Can you work these out from the model? Positions are in its coordinate system, mm. A direction names the side the tool comes from. Give positions to 0.01 mm unless a question says otherwise; leave off trailing zeros. Loops run counter-clockwise (first coordinate to the right, second up) from the corner with the lowest first, then second, coordinate; pieces in that order, holes last. Notation, with made-up numbers: (80, 36) -> (124, 36) arc R23 ccw to (124, 50) -> close; hole circle Ø10 at (71.5, -18). An arc over 180 degrees is marked (long way). One line per question, with ' | ' between items.
Autodesk Inventor part; units mm, degrees
ref_plane "YZ Plane" through (0, 0, 0) normal (1, 0, 0) x (0, 1, 0)
ref_plane "XZ Plane" through (0, 0, 0) normal (0, 1, 0) x (-1, 0, 0)
ref_plane "XY Plane" through (0, 0, 0) normal (0, 0, 1) x (1, 0, 0)
sketch "Sketch1" plane through (0, 0, 0) normal (0, 1, 0) x (-1, 0, 0)
  circle A0 centre (0, 0) radius 10
  dimension "d0" = 20
extrude "Extrusion1" add sketch "Sketch1" along normal blind 125
thread "Thread1"
sketch "Sketch2" plane through (0, 0, 0) normal (0, -1, 0) x (1, 0, 0)
  circle A0 centre (0, 0) radius 6
  dimension "d5" = 12
extrude "Extrusion2" add sketch "Sketch2" along normal blind 55
fillet "Fillet1" radius 0.5 2 edges at (-6, -55, 0) (10, 125, 0)
properties part number "LeadScrew" material "Steel, Alloy"
Q1. For pin 1 Ø1.5 at (x, y) = (-5, 7.5) entering from -Z; pin 2 Ø10 at (x, y) = (-4, 29) entering from -Z; pin 3 Ø3 at (x, y) = (4, 60) entering from -Z; pin 4 Ø4 at (y, z) = (82, -3.5) entering from -X, each with a flat end and sliding along its axis, tell me the tip position at first contact or that it passes through.
Entries:
pin 1: z = -9.05 | pin 2: z = -10 | pin 3: z = -9.68 | pin 4: x = -9.89
Q2. If we section it at B-B (x = 0): Write out the boundary of the cut face in (y, z).
Entries:
outline: (-55, -5.5) arc R0.5 ccw to (-54.5, -6) -> (0, -6) -> (0, -10) -> (124.5, -10) arc R0.5 ccw to (125, -9.5) -> (125, 9.5) arc R0.5 ccw to (124.5, 10) -> (0, 10) -> (0, 6) -> (-54.5, 6) arc R0.5 ccw to (-55, 5.5) -> close
Q3. If we section it at C-C (y = 81): Write out the boundary of the cut face in (x, z).
Entries:
outline: circle Ø20 at (0, 0)
Q4. On a 3-axis mill with a long thin cutter (end or side, diameter ignored), from which of +Z, -Z, +X, -X, +Y, -Y can I reach the whole of each face in a straight line? I mean faces 1 (the face through (-6, -27, 0)), 2 (the face through (0, 125, 0)). Say none if no direction works.
Entries:
face 1: -Y | face 2: +Z, -Z, +X, -X, +Y
Q5. If I drill on probe 1 along Y at (x, z) = (0.25, -6.75); probe 2 along X at (y, z) = (-42.5, -0.5); probe 3 along X at (y, z) = (9, 1.75), over which ranges is the centre line in solid material (lowest first)? Write a range as from..to.
Entries:
probe 1: 0..125 | probe 2: -5.98..5.98 | probe 3: -9.85..9.85
Q6. If we section it at A-A (z = 0): Write out the boundary of the cut face in (x, y).
Entries:
outline: (-10, 0) -> (-6, 0) -> (-6, -54.5) arc R0.5 ccw to (-5.5, -55) -> (5.5, -55) arc R0.5 ccw to (6, -54.5) -> (6, 0) -> (10, 0) -> (10, 124.5) arc R0.5 ccw to (9.5, 125) -> (-9.5, 125) arc R0.5 ccw to (-10, 124.5) -> close
